```python
from build123d import *

# Parameters (mm, degrees)
PAD_DEPTH    = 140
PAD001_DEPTH = 140


with BuildPart() as part:
    # Sketch → Pad (new body)
    with BuildSketch(Plane.XZ):
        Polygon((1.709151, 14), (0.847738, 14), (0.847738, 15), (2.609062, 15), (2.609062, 12.991093), (1, 11.170912), (1, 1.090989), (14, 1.090989), (14, 11.170912), (12.390938, 12.991093), (12.390938, 15), (14.152262, 15), (14.152262, 14), (13.290849, 14), (13.290849, 13.145577), (15, 11.212176), (15, 0), (0, 0), (0, 11.212176), (1.709151, 13.145577), align=None)
    extrude(amount=PAD_DEPTH)

    # Sketch001 → Pad001 (join)
    with BuildSketch(Plane.XZ):
        Polygon((1.670899, 13.98237), (0.833981, 13.98237), (0.833981, 15.0478), (14.219909, 15.0478), (14.219909, 13.970164), (13.277989, 13.970164), (13.277989, 13.140446), (14.96773, 13.140446), (14.96773, 15.855778), (0.035527, 15.855778), (0.035527, 13.198529), (1.670899, 13.198529), align=None)
    extrude(amount=PAD001_DEPTH)


solid = part.part
```
Check sheet for the modelled part. Datum: model origin and axes. Units: mm. A direction names the side the tool comes from. Round coordinates to 2 decimals unless told otherwise and drop trailing zeros. Loops run counter-clockwise (first coordinate to the right, second up) from the corner with the lowest first, then second, coordinate; pieces in that order, holes last. Notation, with made-up numbers: (35.25, -12.5) - (39.25, -12.5) arc R25 cw to (39.25, 22.5) - close; hole circle Ø2 at (-34, 60). An arc over 180 degrees is marked (long way). Answer as a JSON object with one key per item and string values. Group by question number.
Q1. Mould release check, pull along Z, two halves, no side actions. Record for faces 3 (the face through (0.7, 0, 8)), 4 (the face through (7, -69, 15.048)), 5 (the face through (8, -69, 0)): released by +Z, released by -Z, zero draft, split by the parting line, or undercut.
Q2. Scan lines: line 1 along X through (y, z) = (-120, 4.5); line 2 along Z through (x, y) = (7.5, -26.5); line 3 along X through (y, z) = (-108, 12.5). Record each from-to range of solid material in increasing order. Write a range as [from, to].
Q3. Set-up check for faces 1 (the face through (0, -69, 6)), 2 (the face through (7, -69, 1.091)): record each of +Z, -Z, +X, -X, +Y, -Y from which the full face is reachable in a straight line by a thin tool's end or side.
Q4. Gauge pin test, flat ends, axial feed: P1, Ø0.8, axis at y = -83, z = 14, coming from the +X side; P2, Ø0.9, axis at x = 14, y = -53, coming from the -Z side; P3, Ø0.5, axis at y = -104.5, z = 14.5, coming from the -X side; P4, Ø1.5, axis at x = 9.5, z = 12.5, coming from the +Y side. Record the tip position at first contact, or that the pin passes through.
Q5. Sectioned sample at B-B, the plane x = 6.25. Enter the section's corners in (y, z).
Q6. Sectioned sample at A-A, the plane z = 4.5. Enter the section's corners in (x, y), plus the area to 3 significant figures.
Solution:
{
 "1": {"face 3": "zero draft", "face 4": "undercut", "face 5": "released by -Z"},
 "2": {"line 1": "x = [0, 1], [14, 15]", "line 2": "z = [0, 1.09], [15.05, 15.86]", "line 3": "x = [1.14, 2.17], [12.83, 13.86]"},
 "3": {"face 1": "+Z, -Z, -X, +Y, -Y", "face 2": "+Y, -Y"},
 "4": {"P1": "stops at x = 14.97", "P2": "stops at z = 0", "P3": "stops at x = 0.04", "P4": "passes through"},
 "5": {"outline": "(-140, 0) - (0, 0) - (0, 1.09) - (-140, 1.09) - close; (-140, 15.05) - (0, 15.05) - (0, 15.86) - (-140, 15.86) - close"},
 "6": {"outline": "(0, -140) - (1, -140) - (1, 0) - (0, 0) - close; (14, -140) - (15, -140) - (15, 0) - (14, 0) - close", "area": "280 mm²"}
}
